```python
from build123d import *

# Parameters (mm, degrees)
F1_DEPTH = 200
F2_DEPTH = 10
F3_DEPTH = 30
F0_W     = 20
F0_H     = 60
F4_DEPTH = 60
F5_DEPTH = 90
F6_DEPTH = 120
F7_DEPTH = 150
F8_DEPTH = 180
F9_DEPTH = 210


with BuildPart() as f1:
    # F0 (on Front) → F1 (new body)
    with BuildSketch(Plane.XZ):
        Polygon((120, 100), (-120, 100), (-120, 30), (-105, 30), (-105, 85), (105, 85), (105, -85), (-105, -85), (-105, -30), (-120, -30), (-120, -100), (120, -100), align=None)
    extrude(amount=F1_DEPTH)

    # F1_face (on face) → F2 (join, symmetric)
    with BuildSketch(Plane(origin=(8.881579, 0, 0), x_dir=(1, 0, 0), z_dir=(0, 1, 0))):
        Polygon((-128.881579, -100), (111.118421, -100), (111.118421, 100), (-128.881579, 100), (-128.881579, 30), (-113.881579, 30), (-113.881579, 85), (96.118421, 85), (96.118421, -85), (-113.881579, -85), (-113.881579, -30), (-128.881579, -30), align=None)
    extrude(amount=F2_DEPTH, both=True)

    # F0 (on Front) → F3 (join)
    with BuildSketch(Plane.XZ):
        Polygon((-105, 30), (-120, 30), (-125, 30), (-125, -30), (-120, -30), (-105, -30), align=None)
    extrude(amount=F3_DEPTH)

    # F0 (on Front) → F4 (join)
    with BuildSketch(Plane.XZ):
        with Locations((-135, 0)):
            Rectangle(F0_W, F0_H)
    extrude(amount=F4_DEPTH)

    # F0 (on Front) → F5 (join)
    with BuildSketch(Plane.XZ):
        with Locations((-155, 0)):
            Rectangle(F0_W, F0_H)
    extrude(amount=F5_DEPTH)

    # F0 (on Front) → F6 (join)
    with BuildSketch(Plane.XZ):
        with Locations((-175, 0)):
            Rectangle(F0_W, F0_H)
    extrude(amount=F6_DEPTH)

    # F0 (on Front) → F7 (join)
    with BuildSketch(Plane.XZ):
        with Locations((-195, 0)):
            Rectangle(F0_W, F0_H)
    extrude(amount=F7_DEPTH)

    # F0 (on Front) → F8 (join)
    with BuildSketch(Plane.XZ):
        with Locations((-215, 0)):
            Rectangle(F0_W, F0_H)
    extrude(amount=F8_DEPTH)

    # F0 (on Front) → F9 (join)
    with BuildSketch(Plane.XZ):
        with Locations((-235, 0)):
            Rectangle(F0_W, F0_H)
    extrude(amount=F9_DEPTH)


solid = f1.part
```
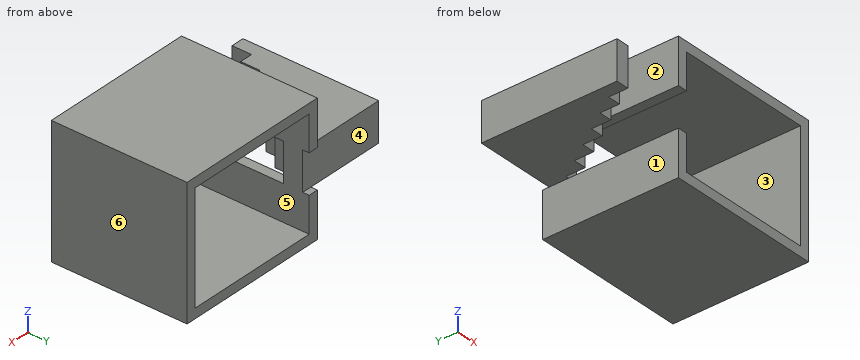
Build history of the part. All positions in model axes, mm. Face numbers are marked on the shaded views. A direction names the side the tool comes from. Round coordinates to 2 decimals unless told otherwise and drop trailing zeros. Write each loop counter-clockwise with the first axis right and the second up, starting at its lowest first coordinate (ties: lowest second). Pieces come first, ordered by that corner, then holes.
1) 3-axis set-ups, long thin cutter, end or side, ignore diameter. For the marked faces 1, 2 and 3: which of +Z, -Z, +X, -X, +Y, -Y reach the whole face in a straight line?
2) Drill centre lines: probe 1 along Z at (x, y) = (-33, -32.5); probe 2 along X at (y, z) = (-135, 38); probe 3 along X at (y, z) = (-24.5, 5.5). Where is each one in solid material? Low to high.
3) Band-saw the part on C-C, the plane x = -13. List the corners of the cut face in (y, z).
4) Band-saw the part on B-B, the plane y = -95. List the corners of the cut face in (x, z).
5) Band-saw the part on A-A, the plane z = -48. List the corners of the cut face in (x, y), and give its area (3 significant figures).
6) Band-saw the part on D-D, the plane y = -6. List the corners of the cut face in (x, z), and give its area (3 significant figures).
7) Mould opens along X. For the marked faces 4, 5 and 6 say: +X half, -X half, draft (parallel to the pull), parting line (faces both ways), or undercut.
8) Pin check, flat tips, straight feed: pin 1 (1 mm diameter, centred on y = -64, z = 37, fed in from -X); pin 2 (8 mm diameter, centred on x = -136.5, z = 27, fed in from -Y); pin 3 (6 mm diameter, centred on x = -152, z = 11.5, fed in from -Y). Stop position of each tip, or through.
Ans:
1. face 1: -Z, -X, +Y, -Y
1. face 2: +Z, -X, +Y, -Y
1. face 3: +Y, -Y
2. probe 1: z = -100 to -85, 85 to 100
2. probe 2: x = -120 to -105, 105 to 120
2. probe 3: x = -245 to -105, 105 to 120
3. outline: (-200, -100) - (10, -100) - (10, -85) - (-200, -85) - close; (-200, 85) - (10, 85) - (10, 100) - (-200, 100) - close
4. outline: (-245, -30) - (-165, -30) - (-165, 30) - (-245, 30) - close; (-120, -100) - (120, -100) - (120, 100) - (-120, 100) - (-120, 30) - (-105, 30) - (-105, 85) - (105, 85) - (105, -85) - (-105, -85) - (-105, -30) - (-120, -30) - close
5. outline: (-120, -200) - (-105, -200) - (-105, 10) - (-120, 10) - close; (105, -200) - (120, -200) - (120, 10) - (105, 10) - close
5. area: 6,300 mm2
6. outline: (-245, -30) - (-120, -30) - (-120, -100) - (120, -100) - (120, 100) - (-120, 100) - (-120, 30) - (-245, 30) - close; hole (-105, -85) - (105, -85) - (105, 85) - (-105, 85) - close
6. area: 19,800 mm2
7. face 4: draft
7. face 5: undercut
7. face 6: +X half
8. pin 1: stops at x = -120
8. pin 2: stops at y = -60
8. pin 3: stops at y = -90
